Part print with two shaded views. Sizes in mm from the minimum x, y, z corner. A direction names the side the tool comes from. Coordinates: 2 decimals unless noted, no trailing zeros. Loops run counter-clockwise (first coordinate to the right, second up) from the corner with the lowest first, then second, coordinate; pieces in that order, holes last.
(1) Slice it at A-A (x = 20.5). Give the cut face in (y, z).
(2) Slice it at B-B (z = 4.5). Give the cut face in (x, y).
(3) Wall check: L1, parallel to X at y = 1.25, z = 2.5. Give the ranges that are in metal, low to high.
(4) Flat gauge pins, fed straight in: P1, Ø0.5, axis at y = 0.5, z = 20, coming from the +X side; P2, Ø8, axis at x = 22, z = 26, coming from the -Y side; P3, Ø0.9, axis at x = 23, y = 0.5, coming from the -Z side; P4, Ø0.5, axis at x = 5.5, y = 1, coming from the -Z side. Where does each tip first touch, or does it go through?
(5) Slice it at C-C (y = 0.95). Give the number of separate pieces and of enclosed holes in the cut face, and give its area (3 significant figures).
(6) Tool access for the marked faces 1 and 2: list every direction of +Z, -Z, +X, -X, +Y, -Y with a clear straight run to the whole face (end or side of a thin tool).
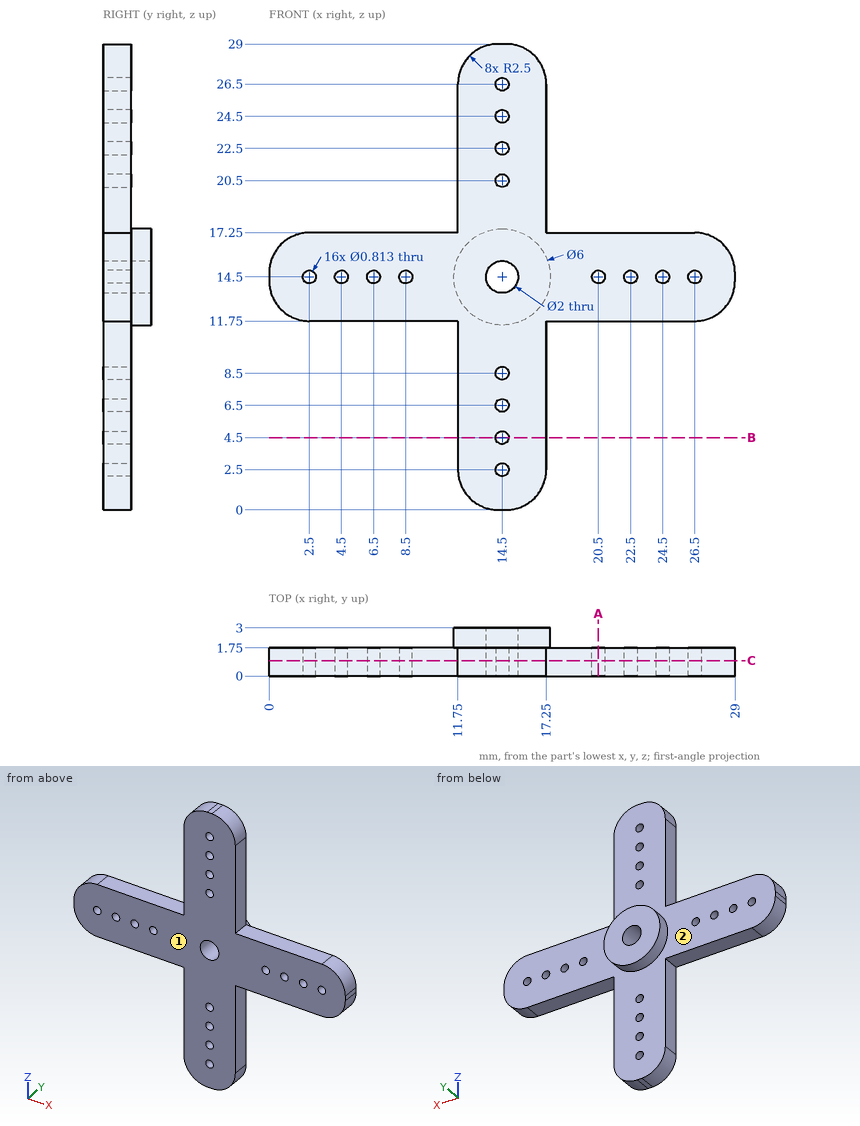
Response values:
1. outline: (0, 11.75) - (1.75, 11.75) - (1.75, 14.09) - (0, 14.09) - close; (0, 14.91) - (1.75, 14.91) - (1.75, 17.25) - (0, 17.25) - close
2. outline: (11.75, 0) - (14.09, 0) - (14.09, 1.75) - (11.75, 1.75) - close; (14.91, 0) - (17.25, 0) - (17.25, 1.75) - (14.91, 1.75) - close
3. L1: x = 11.75 to 14.09, 14.91 to 17.25
4. P1: stops at x = 17.25
4. P2: passes through
4. P3: stops at z = 11.75
4. P4: stops at z = 11.75
5. separate pieces: 1
5. enclosed holes: 17
5. area: 267 mm2
6. face 1: +Z, -Z, +X, -X, -Y
6. face 2: +Y
